```python
from build123d import *

# Parameters (mm, degrees)
SKETCH_1_W          = 42
SKETCH_1_H          = 42
EXTRUDE_1_DEPTH     = 25
SKETCH_2_W          = 38
SKETCH_2_H          = 38
CUT_EXTRUDE_1_DEPTH = 22
SKETCH_3_R          = 9.25
CUT_EXTRUDE_2_DEPTH = 65.443773943
SKETCH_4_W          = 15
SKETCH_4_H          = 10
EXTRUDE_2_DEPTH     = 30
SKETCH_5_W          = 27
SKETCH_5_H          = 12
CUT_EXTRUDE_3_DEPTH = 2
SKETCH_6_W          = 27
SKETCH_6_H          = 13
CUT_EXTRUDE_4_DEPTH = 2
FILLET_1_R          = 2


with BuildPart() as part:
    # 스케치1 → 보스-돌출1 (new body)
    with BuildSketch(Plane.XY):
        with Locations((21, -21)):
            Rectangle(SKETCH_1_W, SKETCH_1_H)
    extrude(amount=EXTRUDE_1_DEPTH)

    # 스케치2 → 컷-돌출1 (cut)
    with BuildSketch(Plane.XY.offset(25)):
        with Locations((21, -21)):
            Rectangle(SKETCH_2_W, SKETCH_2_H)
    extrude(amount=-CUT_EXTRUDE_1_DEPTH, mode=Mode.SUBTRACT)

    # 스케치3 → 컷-돌출2 (cut, through all)
    with BuildSketch(Plane(origin=(0, 0, 0), x_dir=(-1, 0, 0), z_dir=(0, 0, -1))):
        with Locations((-21, -21)):
            Circle(SKETCH_3_R)
    extrude(amount=-CUT_EXTRUDE_2_DEPTH, mode=Mode.SUBTRACT)

    # 스케치4 → 보스-돌출2 (add)
    with BuildSketch(Plane.ZY):
        with Locations((17.5, -21)):
            Rectangle(SKETCH_4_W, SKETCH_4_H)
    extrude(amount=EXTRUDE_2_DEPTH)

    # 스케치5 → 컷-돌출3 (cut)
    with BuildSketch(Plane.XZ.offset(26)):
        with Locations((-15.5, 19)):
            Rectangle(SKETCH_5_W, SKETCH_5_H)
    extrude(amount=-CUT_EXTRUDE_3_DEPTH, mode=Mode.SUBTRACT)

    # 스케치6 → 컷-돌출4 (cut)
    with BuildSketch(Plane(origin=(0, -16, 0), x_dir=(1, 0, 0), z_dir=(0, 1, 0))):
        with Locations((-15.5, -18.5)):
            Rectangle(SKETCH_6_W, SKETCH_6_H)
    extrude(amount=-CUT_EXTRUDE_4_DEPTH, mode=Mode.SUBTRACT)

    # 필렛1
    fillet_1_edges = [part.edges().sort_by_distance(p)[0] for p in [
        (0, -26, 17.5),
        (0, -16, 17.5),
    ]]
    fillet(fillet_1_edges, radius=FILLET_1_R)


solid = part.part
```
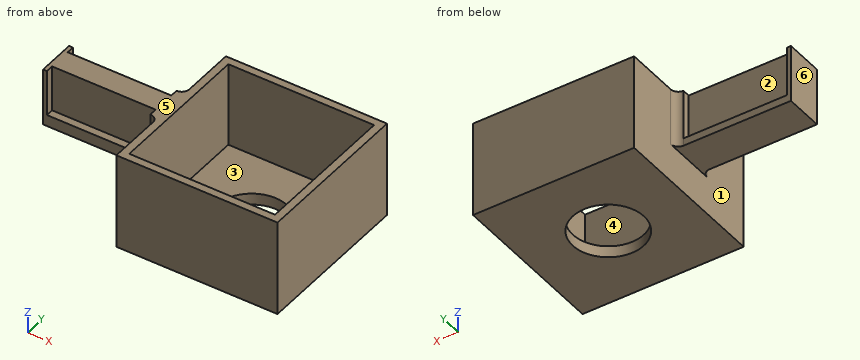
Check sheet for the modelled part. Datum: model origin and axes. Units: mm. Face numbers are marked on the shaded views. A direction names the side the tool comes from. Give positions to 0.01 mm unless a question says otherwise; leave off trailing zeros. Write each loop counter-clockwise with the first axis right and the second up, starting at its lowest first coordinate (ties: lowest second). Pieces come first, ordered by that corner, then holes.
Item 1: Cross-section at B-B (y = -21). Enter the section's corners in (x, z).
Item 2: Gauge pin test, flat ends, axial feed: pin 1 (1 mm diameter, centred on x = -9.5, y = -25.5, fed in from +Z); pin 2 (6 mm diameter, centred on y = -30, z = 9.5, fed in from -X); pin 3 (24 mm diameter, centred on x = 21, y = -21, fed in from +Z). Record the tip position at first contact, or that the pin passes through.
Item 3: Draft check along X on the marked faces 4, 5 and 6. Enter one of: released by +X, released by -X, zero draft, split by the parting line, or undercut.
Item 4: Access from +Z, -Z, +X, -X, +Y, -Y to the whole of each face (thin tool, end or side, straight path). Record for the marked faces 1, 2 and 3.
Item 5: Cross-section at C-C (z = 14.75). Enter the section's corners in (x, y).
Item 6: Scan lines: L1, parallel to X at y = -19.5, z = 22.75; L2, parallel to X at y = -5.5, z = 16.25; L3, parallel to Y at x = 37, z = 22.25. Record each from-to range of solid material in increasing order.
Item 7: Cross-section at D-D (x = -16). Enter the section's corners in (y, z), and give its area (3 significant figures).
Item 8: Cross-section at A-A (x = 21). Enter the section's corners in (y, z), and give its area (4 significant figures).
Report:
1. outline: (-30, 10) - (0, 10) - (0, 0) - (11.75, 0) - (11.75, 3) - (2, 3) - (2, 25) - (-30, 25) - close; (30.25, 0) - (42, 0) - (42, 25) - (40, 25) - (40, 3) - (30.25, 3) - close
2. pin 1: stops at z = 13
2. pin 2: stops at x = -0.24
2. pin 3: stops at z = 3
3. face 4: undercut
3. face 5: zero draft
3. face 6: released by -X
4. face 1: -Z, -X
4. face 2: +Z, +Y
4. face 3: +Z
5. outline: (-30, -26) - (-29, -26) - (-29, -24) - (-2, -24) - (-2, -26) arc R2 cw to (0, -28) - (0, -42) - (42, -42) - (42, 0) - (0, 0) - (0, -14) arc R2 cw to (-2, -16) - (-2, -18) - (-29, -18) - (-29, -16) - (-30, -16) - close; hole (2, -40) - (40, -40) - (40, -2) - (2, -2) - close
6. L1: x = -30 to 2, 40 to 42
6. L2: x = 0 to 2, 40 to 42
6. L3: y = -42 to -40, -2 to 0
7. outline: (-26, 10) - (-16, 10) - (-16, 12) - (-18, 12) - (-18, 25) - (-24, 25) - (-24, 13) - (-26, 13) - close
7. area: 100 mm2
8. outline: (-42, 0) - (-30.25, 0) - (-30.25, 3) - (-40, 3) - (-40, 25) - (-42, 25) - close; (-11.75, 0) - (0, 0) - (0, 25) - (-2, 25) - (-2, 3) - (-11.75, 3) - close
8. area: 158.5 mm2
